Input: part model. Units: mm. Frame: model coordinates. A direction names the side the tool comes from. Coordinates: 2 decimals unless noted, no trailing zeros. Order: outer loops, then holes, each group sorted by start corner. A loop starts at its lowest first (then second) coordinate and runs counter-clockwise, first axis right, second up. Notation, with made-up numbers: (30, -25.5) -> (58, -25.5) arc R19 cw to (58, 0.5) -> close; hole circle Ø2 at (27, 11.5). An arc over 180 degrees is marked (long way). Use one line per item in the form item = value. Start each with the question number.
1) Section query A-A on y = 3.2. Output: boundary loops of the cut face in (x, z), then the cut area to 3 significant figures.
2) Ray query, line 1 along X through (y, z) = (1.8, 0.8); line 2 along Z through (x, y) = (5.75, 1.45); line 3 along Y through (x, z) = (5.5, 0.9). Return the intervals inside material, ascending.
3) Pin query (flat end, axial travel): pin 1 (1.1 mm diameter, centred on y = 1, z = 0.5, fed in from -X); pin 2 (1 mm diameter, centred on x = 0, y = 1.5, fed in from -Z). Return the tip coordinate at first contact, or that it passes through.
4) Section query C-C on y = 1.4. Output: boundary loops of the cut face in (x, z) (3 decimals), then the cut area to 4 significant figures.
5) Section query B-B on z = 0.4. Output: boundary loops of the cut face in (x, y), then the cut area to 3 significant figures.
6) Draft query along X for faces 1 (the cylindrical face through (1.79, 0.98, -0.25)), 2 (the cylindrical face through (5.243, 1.563, -0.246)), 3 (the flat face through (3, -1, 1)), 4 (the flat face through (3.25, -0.7, 0.5)). Return one class per face: pulls with the +X half, pulls with the -X half, needs draft (parallel to the pull), parting line crosses it, or undercut.
7) Section query D-D on x = 4. Output: boundary loops of the cut face in (y, z).
8) Access query for faces 5 (the flat face through (1.95, -0.7, 0.5)), 6 (the flat face through (1.8, 1.4, -0.5)). Directions: +Z, -Z, +X, -X, +Y, -Y. A direction counts if a zero-diameter tool reaches every point of the face in a straight line with its end or side. Return the directions, or none.
from build123d import *

# Parameters (mm, degrees)
F0_W     = 6.7
F0_H     = 2.8
F1_DEPTH = 1.35
F2_W     = 0.4
F2_H     = 0.992101
F2_H_2   = 1.01787
F2_H_3   = 1.082292
F2_W_2   = 0.883373
F2_H_4   = 0.45
F2_W_3   = 0.808923
F2_W_4   = 0.892466
F2_W_5   = 0.931122
F3_DEPTH = 0.15
F4_W     = 1.3
F4_H     = 1.35
F5_DEPTH = 1
F6_R     = 0.425
F7_DEPTH = 0.5


with BuildPart() as f1:
    # F0 (on Top) → F1 (new body)
    with BuildSketch(Plane.XY):
        with Locations((3.35, 1.4)):
            Rectangle(F0_W, F0_H)
    extrude(amount=F1_DEPTH)

    # F2 (on Top) → F3 (join)
    with BuildSketch(Plane.XY):
        with Locations((5.5, 3.29605)):
            Rectangle(F2_W, F2_H)
        with Locations((4.1, 3.308935)):
            Rectangle(F2_W, F2_H_2)
        with Locations((1.2, 3.341146)):
            Rectangle(F2_W, F2_H_3)
        with Locations((7.141686, 2.575)):
            Rectangle(F2_W_2, F2_H_4)
        with Locations((7.104461, 0.225)):
            Rectangle(F2_W_3, F2_H_4)
        with Locations((-0.446233, 2.575)):
            Rectangle(F2_W_4, F2_H_4)
        with Locations((-0.465561, 0.225)):
            Rectangle(F2_W_5, F2_H_4)
    extrude(amount=F3_DEPTH)

    # F4 (on Top) → F5 (join)
    with BuildSketch(Plane.XY):
        with Locations((2.6, -0.675)):
            Rectangle(F4_W, F4_H)
    extrude(amount=F5_DEPTH)

    # F6 (on face) → F7 (join)
    with BuildSketch(Plane(origin=(0, 0, 0), x_dir=(1, 0, 0), z_dir=(0, 0, -1))):
        with Locations((4.85, -1.4)):
            Circle(F6_R)
        with Locations((1.85, -1.4)):
            Circle(F6_R)
    extrude(amount=F7_DEPTH)


solid = f1.part
Answers below:
q1.outline = (1, 0) -> (1.4, 0) -> (1.4, 0.15) -> (1, 0.15) -> close; (3.9, 0) -> (4.3, 0) -> (4.3, 0.15) -> (3.9, 0.15) -> close; (5.3, 0) -> (5.7, 0) -> (5.7, 0.15) -> (5.3, 0.15) -> close
q1.area = 0.180 mm^2
q2.line_1 = 0 to 6.7
q2.line_2 = 0 to 1.35
q2.line_3 = 0 to 2.8
q3.pin_1 = 0
q3.pin_2 = 0
q4.outline = (0, 0) -> (1.425, 0) -> (1.425, -0.5) -> (2.275, -0.5) -> (2.275, 0) -> (4.425, 0) -> (4.425, -0.5) -> (5.275, -0.5) -> (5.275, 0) -> (6.7, 0) -> (6.7, 1.35) -> (0, 1.35) -> close
q4.area = 9.895 mm^2
q5.outline = (0, 0) -> (1.95, 0) -> (1.95, -1.35) -> (3.25, -1.35) -> (3.25, 0) -> (6.7, 0) -> (6.7, 2.8) -> (0, 2.8) -> close
q5.area = 20.5 mm^2
q6.face_1 = undercut
q6.face_2 = undercut
q6.face_3 = needs draft
q6.face_4 = pulls with the +X half
q7.outline = (0, 0) -> (3.82, 0) -> (3.82, 0.15) -> (2.8, 0.15) -> (2.8, 1.35) -> (0, 1.35) -> close
q8.face_5 = +Z, -Z, -X, -Y
q8.face_6 = -Z, +X, -X, +Y, -Y
